```python
from build123d import *

# Parameters (mm, degrees)
EXTRUDE_THIN1_DEPTH = 584.2
BOSS_EXTRUDE1_START = 177.8
BOSS_EXTRUDE1_DEPTH = 177.8
SKETCH4_W           = 482.6
SKETCH4_H           = 6.35
BOSS_EXTRUDE2_DEPTH = 31.75


with BuildPart() as part:
    # Sketch1 → Extrude-Thin1 (new, symmetric)
    with BuildSketch(Plane.XY):
        with BuildLine():
            Line((-206.6, -79.375), (-111.35, -79.375))
            ThreePointArc((-111.35, -79.375), (-104.614807909, -76.585192091), (-101.825, -69.85))
            Line((-101.825, -69.85), (-101.825, -6.35))
            ThreePointArc((-101.825, -6.35), (-100.89506403, -4.10493597), (-98.65, -3.175))
            Line((-98.65, -3.175), (98.65, -3.175))
            ThreePointArc((98.65, -3.175), (100.89506403, -4.10493597), (101.825, -6.35))
            Line((101.825, -6.35), (101.825, -69.85))
            ThreePointArc((101.825, -69.85), (104.614807909, -76.585192091), (111.35, -79.375))
            Line((111.35, -79.375), (206.6, -79.375))
            Line((206.6, -79.375), (206.6, -73.025))
            Line((206.6, -73.025), (111.35, -73.025))
            ThreePointArc((111.35, -73.025), (109.10493597, -72.09506403), (108.175, -69.85))
            Line((108.175, -69.85), (108.175, -6.35))
            ThreePointArc((108.175, -6.35), (105.385192091, 0.385192091), (98.65, 3.175))
            Line((98.65, 3.175), (-98.65, 3.175))
            ThreePointArc((-98.65, 3.175), (-105.385192091, 0.385192091), (-108.175, -6.35))
            Line((-108.175, -6.35), (-108.175, -69.85))
            ThreePointArc((-108.175, -69.85), (-109.10493597, -72.09506403), (-111.35, -73.025))
            Line((-111.35, -73.025), (-206.6, -73.025))
            Line((-206.6, -73.025), (-206.6, -79.375))
        make_face()
    extrude(amount=EXTRUDE_THIN1_DEPTH, both=True)

    # Sketch3 → Boss-Extrude1 (add)
    with BuildSketch(Plane.XY.offset(584.2).offset(BOSS_EXTRUDE1_START)):
        with BuildLine():
            Line((-108.175, -69.85), (-101.825, -69.85))
            Line((-101.825, -69.85), (-101.825, -6.35))
            ThreePointArc((-101.825, -6.35), (-100.89506403, -4.10493597), (-98.65, -3.175))
            Line((-98.65, -3.175), (98.65, -3.175))
            ThreePointArc((98.65, -3.175), (100.89506403, -4.10493597), (101.825, -6.35))
            Line((101.825, -6.35), (101.825, -69.85))
            Line((101.825, -69.85), (108.175, -69.85))
            Line((108.175, -69.85), (108.175, -6.35))
            ThreePointArc((108.175, -6.35), (105.385192091, 0.385192091), (98.65, 3.175))
            Line((98.65, 3.175), (-98.65, 3.175))
            ThreePointArc((-98.65, 3.175), (-105.385192091, 0.385192091), (-108.175, -6.35))
            Line((-108.175, -6.35), (-108.175, -69.85))
        make_face()
    boss_extrude1 = extrude(amount=-BOSS_EXTRUDE1_DEPTH)

    # Sketch4 → Boss-Extrude2 (add)
    with BuildSketch(Plane(origin=(206.6, 0, 0), x_dir=(0, 0, -1), z_dir=(1, 0, 0))):
        with Locations((0, -76.2)):
            Rectangle(SKETCH4_W, SKETCH4_H)
    boss_extrude2 = extrude(amount=BOSS_EXTRUDE2_DEPTH)

    # Mirror1: Boss-Extrude1 across plane
    add(boss_extrude1.mirror(Plane.XY))

    # Mirror2: Boss-Extrude2 across plane
    add(boss_extrude2.mirror(Plane(origin=(0, 0, 0), x_dir=(0, 0, 1), z_dir=(1, 0, 0))))


solid = part.part
```
Can you work these out from the model? Positions are in its coordinate system, mm. A direction names the side the tool comes from. Coordinates: 2 decimals unless noted, no trailing zeros. Order: outer loops, then holes, each group sorted by start corner. A loop starts at its lowest first (then second) coordinate and runs counter-clockwise, first axis right, second up.
1. If we section it at A-A (y = -34): Please give me the cut outline in (x, z) (3 decimals), then the cut area to 3 significant figures.
2. If we section it at D-D (z = 522): Please give me the cut outline in (x, y) (3 decimals), then the cut area to 3 significant figures.
3. Thinking about a two-plate mould opening in X: for faces 1 (the face through (101.825, -38, -11)), 2 (the face through (160, -79.375, 8)), 3 (the face through (-108.175, -38, -11)), which applies, +X half, -X half, draft (parallel to the pull), parting line (faces both ways), or undercut?
4. I need wall thicknesses on line 1 (X direction, y = -6, z = 387); line 2 (Y direction, x = -14, z = 61.5) (3 decimals); line 3 (Y direction, x = -173, z = -152) (3 decimals). Which ranges of each line are inside material? Lowest first, please.
5. For faces 4 (the face through (-160, -73.025, 8)), 5 (the face through (-1, -3.175, -11)), 6 (the face through (162, -73.025, 8)), 7 (the face through (-9, -1, 762)), which set-ups out of +Z, -Z, +X, -X, +Y, -Y let a thin tool reach every point of the face, with its end or its side?
6. If we section it at B-B (z = -223): Please give me the cut outline in (x, y) (3 decimals).
7. If we section it at C-C (x = -163): Please give me the cut outline in (y, z) (3 decimals), then the cut area to 3 significant figures.
8. I'm going to push flat-ended pins straight in: pin 1 (10.5 mm diameter, centred on x = -139, y = -74.5, fed in from +Z); pin 2 (1 mm diameter, centred on y = -55.5, z = -495, fed in from +X) (3 decimals); pin 3 (1.9 mm diameter, centred on x = -105, z = -661, fed in from -Y). Where does each tip first touch, or does it pass through?
Entries:
1. outline: (-108.175, -762) - (-101.825, -762) - (-101.825, 762) - (-108.175, 762) - close; (101.825, -762) - (108.175, -762) - (108.175, 762) - (101.825, 762) - close
1. area: 19,400 mm2
2. outline: (-206.6, -79.375) - (-111.35, -79.375) arc R9.525 ccw to (-101.825, -69.85) - (-101.825, -6.35) arc R3.175 cw to (-98.65, -3.175) - (98.65, -3.175) arc R3.175 cw to (101.825, -6.35) - (101.825, -69.85) arc R9.525 ccw to (111.35, -79.375) - (206.6, -79.375) - (206.6, -73.025) - (111.35, -73.025) arc R3.175 cw to (108.175, -69.85) - (108.175, -6.35) arc R9.525 ccw to (98.65, 3.175) - (-98.65, 3.175) arc R9.525 ccw to (-108.175, -6.35) - (-108.175, -69.85) arc R3.175 cw to (-111.35, -73.025) - (-206.6, -73.025) - close
2. area: 3,520 mm2
3. face 1: undercut
3. face 2: draft
3. face 3: -X half
4. line 1: x = -108.17 to -101.81, 101.81 to 108.17
4. line 2: y = -3.175 to 3.175
4. line 3: y = -79.375 to -73.025
5. face 4: +Z, -Z, -X, +Y
5. face 5: +Z, -Z, -Y
5. face 6: +Z, -Z, +X, +Y
5. face 7: +Z, +X, -X, +Y, -Y
6. outline: (-238.35, -79.375) - (-111.35, -79.375) arc R9.525 ccw to (-101.825, -69.85) - (-101.825, -6.35) arc R3.175 cw to (-98.65, -3.175) - (98.65, -3.175) arc R3.175 cw to (101.825, -6.35) - (101.825, -69.85) arc R9.525 ccw to (111.35, -79.375) - (238.35, -79.375) - (238.35, -73.025) - (111.35, -73.025) arc R3.175 cw to (108.175, -69.85) - (108.175, -6.35) arc R9.525 ccw to (98.65, 3.175) - (-98.65, 3.175) arc R9.525 ccw to (-108.175, -6.35) - (-108.175, -69.85) arc R3.175 cw to (-111.35, -73.025) - (-238.35, -73.025) - close
7. outline: (-79.375, -584.2) - (-73.025, -584.2) - (-73.025, 584.2) - (-79.375, 584.2) - close
7. area: 7,420 mm2
8. pin 1: stops at z = 584.2
8. pin 2: stops at x = 108.175
8. pin 3: stops at y = -69.85
